Check sheet for the modelled part. Datum: model origin and axes. Units: mm. Face numbers are marked on the shaded views. A direction names the side the tool comes from. Round coordinates to 2 decimals unless told otherwise and drop trailing zeros. Loops run counter-clockwise (first coordinate to the right, second up) from the corner with the lowest first, then second, coordinate; pieces in that order, holes last. Notation, with made-up numbers: (-36, -7.5) - (-6, -7.5) arc R25 cw to (-6, 20.5) - close; hole circle Ø11 at (32.5, 66.25). An arc over 180 degrees is marked (long way). Put each result on its own line as item: value.
```python
from build123d import *

# Parameters (mm, degrees)
BOSS_EXTRUDE2_DEPTH = 25
RIB4_REACH          = 82.75
SKETCH2_WALL_W      = 240.282714568
SKETCH2_WALL_H      = 10


with BuildPart() as part:
    # Sketch1 → Boss-Extrude2 (new, symmetric)
    with BuildSketch(Plane.XY):
        Polygon((0, 0), (-61.820224508, 0), (-61.820224508, -12.662921305), (0, -12.662921305), (13.528089841, -12.662921305), (13.528089841, 45.539325687), (0, 45.539325687), align=None)
    extrude(amount=BOSS_EXTRUDE2_DEPTH, both=True)

    # Sketch2 wall → Rib4 (add, up to next)
    with BuildSketch(Plane(origin=(-30.910112254, 22.769662844, 0), x_dir=(-0.805133069987, -0.593094208042, 0), z_dir=(0.593094208042, -0.805133069987, 0)), mode=Mode.PRIVATE) as rib4_sk1:
        Rectangle(SKETCH2_WALL_W, SKETCH2_WALL_H)
    rib4_tool1 = extrude(rib4_sk1.sketch, amount=RIB4_REACH, mode=Mode.PRIVATE) - part.part
    add(rib4_tool1.solids().sort_by_distance((-30.910112254, 22.769662844, 0))[0])


solid = part.part
```
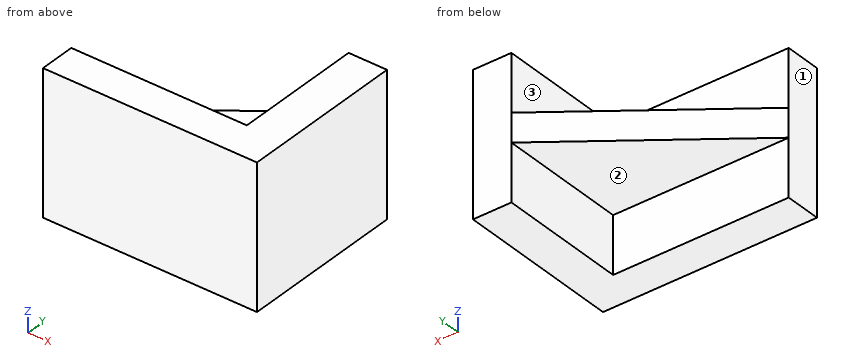
Item 1: Section check C-C on y = 42.5. Enter the section's corners in (x, z).
Filled sheet:
outline: (-4.13, -5) - (0, -5) - (0, -25) - (13.53, -25) - (13.53, 25) - (0, 25) - (0, 5) - (-4.13, 5) - close
Item 2: Go/stop test with flat-tipped pins: pin 1 (6 mm diameter, centred on x = -36.5, y = 4, fed in from +Z); pin 2 (3 mm diameter, centred on x = -15.5, z = 13.5, fed in from +Y); pin 3 (1.5 mm diameter, centred on y = 30, z = 16.5, fed in from -X); pin 4 (4 mm diameter, centred on x = -21, y = 35, fed in from -Z). Record where each tip stops, or that it passes through.
Filled sheet:
pin 1: z = 5
pin 2: y = 0
pin 3: x = 0
pin 4: through
Item 3: Section check A-A on z = 8. Enter the section's corners in (x, y), then the cut area to 3 significant figures.
Filled sheet:
outline: (-61.82, -12.66) - (13.53, -12.66) - (13.53, 45.54) - (0, 45.54) - (0, 0) - (-61.82, 0) - close
area: 1,570 mm²
Item 4: Thickness scan on line 1 (Z direction, x = -0.5, y = 12); line 2 (X direction, y = 14.5, z = -20.5); line 3 (Y direction, x = -23.5, z = -17.5). Record the ranges inside material, lowest first. Write a range as from..to.
Filled sheet:
line 1: -5..5
line 2: 0..13.53
line 3: -12.66..0
Item 5: Section check D-D on z = -3. Enter the section's corners in (x, y).
Filled sheet:
outline: (-61.82, -12.66) - (13.53, -12.66) - (13.53, 45.54) - (0, 45.54) - (-61.82, 0) - close
Item 6: Tool access check on the marked faces 1, 2 and 3. Record the directions out of +Z, -Z, +X, -X, +Y, -Y that give a thin tool (end or side, any length) a straight path to the whole face; none if there is none.
Filled sheet:
face 1: +Z, -Z, -X, +Y, -Y
face 2: -Z, -X, +Y
face 3: +Z, -X, +Y
Item 7: Section check B-B on x = -50. Enter the section's corners in (y, z).
Filled sheet:
outline: (-12.66, -25) - (0, -25) - (0, -5) - (8.71, -5) - (8.71, 5) - (0, 5) - (0, 25) - (-12.66, 25) - close
